The drawing under review shows one solid part. Ordinate dimensions are in mm from its lowest x, y, z. A direction names the side the tool comes from. Give positions to 0.01 mm unless a question says otherwise; leave off trailing zeros. Order: outer loops, then holes, each group sorted by start corner. A loop starts at its lowest first (then second) coordinate and runs counter-clockwise, first axis right, second up. Notation, with made-up numbers: M 43.5,57.25 L 99.5,57.25 A18 cw 99.5,88.25 Z; hole C 53,0 d1. An arc over 180 degrees is marked long. Put each result on its own line as item: value. Start each with the question number.
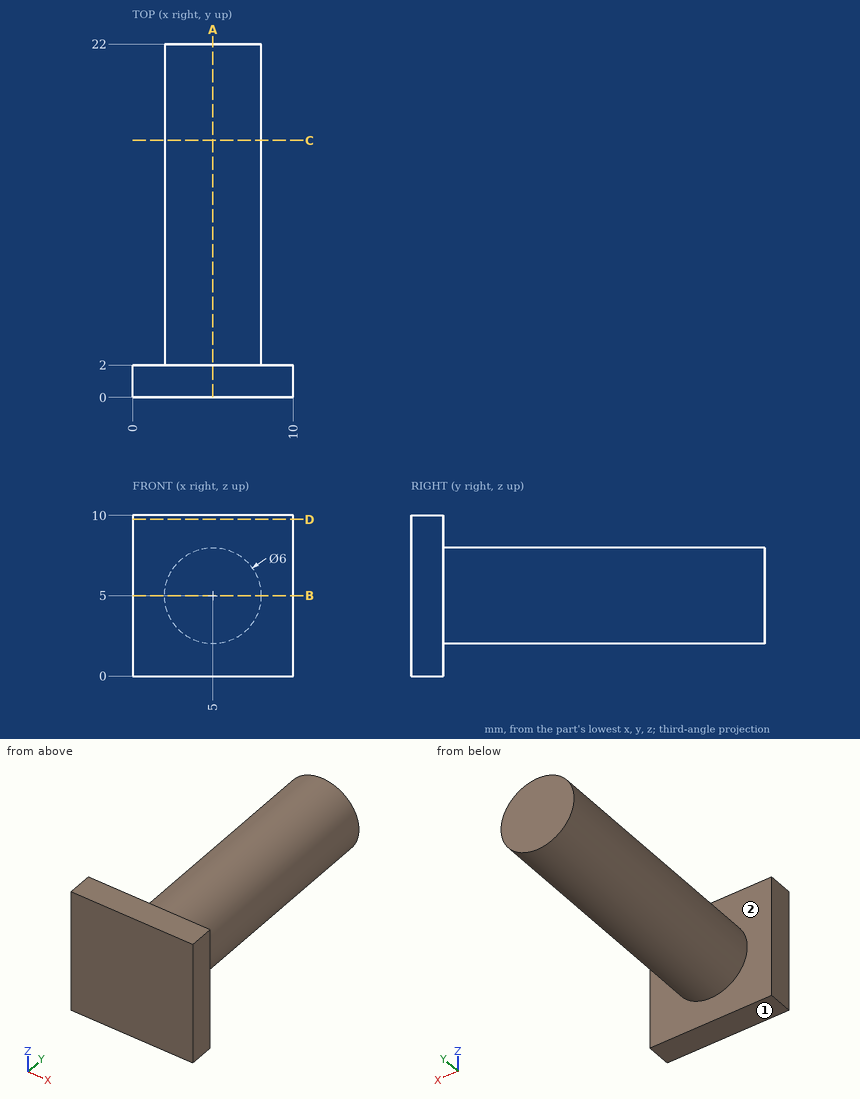
1. Consider section B-B on z = 5. Give the boundary of the cut face in (x, y).
2. Consider section C-C on y = 16. Give the boundary of the cut face in (x, z).
3. Insertion check: pin 1 (5 mm diameter, centred on y = 17, z = 9, fed in from +X); pin 2 (2 mm diameter, centred on x = 2, y = 4.5, fed in from +Z); pin 3 (5 mm diameter, centred on y = 7.5, z = 5, fed in from +X). Each pin has a flat end and moves straight along its axis. Give the tip position at first contact, or say it passes through.
4. Consider section D-D on z = 9.75. Give the boundary of the cut face in (x, y).
5. Machinability: for the marked faces 1 and 2, which of the approach directions +Z, -Z, +X, -X, +Y, -Y give a long, thin tool a straight path to every point of the face, cutting with its end or side? Answer none if there is none.
6. Consider section A-A on x = 5. Give the boundary of the cut face in (y, z), then the cut area to 3 significant figures.
7. To check wall thickness, follow probe 1 along X at (y, z) = (14, 5); probe 2 along Y at (x, z) = (0.5, 9). State the ranges of each line that lie inside material, in increasing order.
Returned:
1. outline: M 0,0 L 10,0 L 10,2 L 8,2 L 8,22 L 2,22 L 2,2 L 0,2 Z
2. outline: C 5,5 d6
3. pin 1: stops at x = 7.6
3. pin 2: stops at z = 7.24
3. pin 3: stops at x = 8
4. outline: M 0,0 L 10,0 L 10,2 L 0,2 Z
5. face 1: -Z, +X, -X, +Y, -Y
5. face 2: +Y
6. outline: M 0,0 L 2,0 L 2,2 L 22,2 L 22,8 L 2,8 L 2,10 L 0,10 Z
6. area: 140 mm2
7. probe 1: x = 2 to 8
7. probe 2: y = 0 to 2
